Geometry: final body of the model. Coordinates: model frame, mm. A direction names the side the tool comes from. Coordinates: 2 decimals unless noted, no trailing zeros. Order: outer loops, then holes, each group sorted by start corner. A loop starts at its lowest first (then second) coordinate and runs counter-clockwise, first axis right, second up. Notation, with made-up numbers: M 4.5,1 L 13.5,1 A24 ccw 13.5,32 Z; hole C 75.5,89.5 d2. An arc over 180 degrees is marked long. Use CSV: the item, a comma, the result in double quotes. Start each with the question number.
Q1. Section query B-B, the plane x = 19. Output: boundary loops of the cut face in (y, z), and give its area (3 significant figures).
Q2. First-contact query: P1, Ø1.6, axis at y = 1, z = 28, coming from the -X side; P2, Ø1, axis at y = 1, z = -6, coming from the +X side; P3, Ø1.6, axis at y = 1.5, z = -24.5, coming from the +X side. Flat tips, straight axial feed; report the tip coordinate or a pass-through.
Q3. Section query C-C, the plane z = 26. Output: boundary loops of the cut face in (x, y), and give its area (3 significant figures).
Q4. Section query A-A, the plane z = 0. Output: boundary loops of the cut face in (x, y), and give its area (4 significant figures).
Q5. Ray query, probe 1 along X at (y, z) = (5.95, 0); probe 2 along X at (y, z) = (0.45, 25); probe 3 along Z at (x, y) = (1, 1.2). Return the intervals inside material, ascending.
Q6. Access query for faces 1 (the face through (-1.978, 1.972, 2.579)), 2 (the face through (19.529, 1.014, 11.275)). Directions: +Z, -Z, +X, -X, +Y, -Y. A direction counts if a zero-diameter tool reaches every point of the face in a straight line with its end or side. Return the directions, or none.
Q7. Section query D-D, the plane z = -19.5. Output: boundary loops of the cut face in (x, y).
Q8. Mould query, pull axis X, two halves, no side actions, for faces 3 (the face through (-8.378, 1.014, 1.435)), 4 (the face through (-2, 6, 0)), 5 (the face through (-5.37, 3.97, -1.19)), 6 (the face through (36.406, 1.014, -6.603)). Classes: +X half, -X half, draft (parallel to the pull), parting line (faces both ways), or undercut.
from build123d import *

# Parameters (mm, degrees)
CROQUIS1_R              = 40
SALIENTE_EXTRUIR1_DEPTH = 2
CROQUIS2_R              = 5.5
SALIENTE_EXTRUIR2_DEPTH = 4
CROQUIS3_R              = 1.75
CORTAR_EXTRUIR1_DEPTH   = 57.885850613
CROQUIS4_R              = 3.25
CORTAR_EXTRUIR2_DEPTH   = 3.5
CHAFL_N1_SIZE           = 2
CORTAR_EXTRUIR3_DEPTH   = 57.709787515


with BuildPart() as part:
    # Croquis1 → Saliente-Extruir1 (new body)
    with BuildSketch(Plane(origin=(0, 0, 0), x_dir=(1, 0, 0), z_dir=(0, 1, 0))):
        with Locations(Location((0, 0, 0), (0, 0, 270))):
            Circle(CROQUIS1_R)
    extrude(amount=SALIENTE_EXTRUIR1_DEPTH)

    # Croquis2 → Saliente-Extruir2 (add)
    with BuildSketch(Plane(origin=(0, 2, 0), x_dir=(1, 0, 0), z_dir=(0, 1, 0))):
        with Locations(Location((0, 0, 0), (0, 0, 270))):
            Circle(CROQUIS2_R)
    extrude(amount=SALIENTE_EXTRUIR2_DEPTH)

    # Croquis3 → Cortar-Extruir1 (cut, through all)
    with BuildSketch(Plane(origin=(0, 6, 0), x_dir=(1, 0, 0), z_dir=(0, 1, 0))):
        with Locations(Location((0, 0, 0), (0, 0, 270))):
            Circle(CROQUIS3_R)
    extrude(amount=-CORTAR_EXTRUIR1_DEPTH, mode=Mode.SUBTRACT)

    # Croquis4 → Cortar-Extruir2 (cut)
    with BuildSketch(Plane(origin=(0, 0, 0), x_dir=(-1, 0, 0), z_dir=(0, -1, 0))):
        with Locations(Location((0, 0, 0), (0, 0, 90))):
            Circle(CROQUIS4_R)
    extrude(amount=-CORTAR_EXTRUIR2_DEPTH, mode=Mode.SUBTRACT)

    # Chaflán1
    # the kernel refuses this chamfer: 2 mm, written as the material it takes off along each edge
    with BuildSketch(Plane(origin=(0, 3.5, 0), x_dir=(0, 0, 1), z_dir=(-1, 0, 0))) as chafl_n1_piece_1_section:
        Polygon((1.75 + CHAFL_N1_SIZE, 0), (1.75, CHAFL_N1_SIZE), (1.75, 0), align=None)
    chafl_n1_piece_1 = revolve(axis=Axis((0, 3.5, 0), (0, 1, 0)), mode=Mode.PRIVATE)
    chafl_n1_piece_1 = chafl_n1_piece_1 & Plane(origin=(0, 4.756379489, 0), x_dir=(0, 0, -1), z_dir=(0, -1, 0)) * Cylinder(3.25, 15, mode=Mode.PRIVATE)
    add(chafl_n1_piece_1, mode=Mode.SUBTRACT)

    # Croquis5 → Cortar-Extruir3 (cut, through all)
    with BuildSketch(Plane(origin=(0, 2, 0), x_dir=(1, 0, 0), z_dir=(0, 1, 0))):
        with BuildLine():
            Line((0, 8.5), (0, 37))
            ThreePointArc((0, 37), (12.654745303, 34.768626969), (23.783141558, 28.343644395))
            Line((23.783141558, 28.343644395), (5.463694682, 6.511377767))
            ThreePointArc((5.463694682, 6.511377767), (2.907171218, 7.987387277), (0, 8.5))
        make_face()
        with BuildLine():
            Line((7.361215932, 4.25), (32.04293994, 18.5))
            ThreePointArc((32.04293994, 18.5), (36.437886861, 6.424982574), (36.437886861, -6.424982574))
            Line((36.437886861, -6.424982574), (8.370865901, -1.47600951))
            ThreePointArc((8.370865901, -1.47600951), (8.370865901, 1.47600951), (7.361215932, 4.25))
        make_face()
        with BuildLine():
            Line((7.361215932, -4.25), (32.04293994, -18.5))
            ThreePointArc((32.04293994, -18.5), (23.783141558, -28.343644395), (12.654745303, -34.768626969))
            Line((12.654745303, -34.768626969), (2.907171218, -7.987387277))
            ThreePointArc((2.907171218, -7.987387277), (5.463694682, -6.511377767), (7.361215932, -4.25))
        make_face()
        with BuildLine():
            Line((0, -8.5), (0, -37))
            ThreePointArc((0, -37), (-12.654745303, -34.768626969), (-23.783141558, -28.343644395))
            Line((-23.783141558, -28.343644395), (-5.463694682, -6.511377767))
            ThreePointArc((-5.463694682, -6.511377767), (-2.907171218, -7.987387277), (0, -8.5))
        make_face()
        with BuildLine():
            Line((-7.361215932, -4.25), (-32.04293994, -18.5))
            ThreePointArc((-32.04293994, -18.5), (-36.437886861, -6.424982574), (-36.437886861, 6.424982574))
            Line((-36.437886861, 6.424982574), (-8.370865901, 1.47600951))
            ThreePointArc((-8.370865901, 1.47600951), (-8.370865901, -1.47600951), (-7.361215932, -4.25))
        make_face()
        with BuildLine():
            Line((-7.361215932, 4.25), (-32.04293994, 18.5))
            ThreePointArc((-32.04293994, 18.5), (-23.783141558, 28.343644395), (-12.654745303, 34.768626969))
            Line((-12.654745303, 34.768626969), (-2.907171218, 7.987387277))
            ThreePointArc((-2.907171218, 7.987387277), (-5.463694682, 6.511377767), (-7.361215932, 4.25))
        make_face()
    extrude(amount=-CORTAR_EXTRUIR3_DEPTH, mode=Mode.SUBTRACT)


solid = part.part
Responses:
1,outline,"M 0,-35.2 L 2,-35.2 L 2,-31.75 L 0,-31.75 Z; M 0,-22.64 L 2,-22.64 L 2,-10.97 L 0,-10.97 Z; M 0,3.35 L 2,3.35 L 2,10.97 L 0,10.97 Z; M 0,31.75 L 2,31.75 L 2,35.2 L 0,35.2 Z"
1,area,"52.4 mm²"
2,P1,"stops at x = -29.33"
2,P2,"stops at x = 39.62"
2,P3,"stops at x = 32.22"
3,outline,"M -30.4,0 L -21.82,0 L -21.82,2 L -30.4,2 Z; M 0,0 L 9.46,0 L 9.46,2 L 0,2 Z; M 26.32,0 L 30.4,0 L 30.4,2 L 26.32,2 Z"
3,area,"44.2 mm²"
4,outline,"M -40,0 L -37,0 L -37,2 L -40,2 Z; M -8.5,0 L -3.25,0 L -3.25,4 L -1.75,5.5 L -1.75,6 L -5.5,6 L -5.5,2 L -8.5,2 Z; M 1.75,5.5 L 3.25,4 L 3.25,0 L 8.5,0 L 8.5,2 L 5.5,2 L 5.5,6 L 1.75,6 Z; M 37,0 L 40,0 L 40,2 L 37,2 Z"
4,area,"54.75 mm²"
5,probe 1,"x = -5.5 to -1.75, 1.75 to 5.5"
5,probe 2,"x = -31.22 to -20.98, 0 to 9.1, 27.28 to 31.22"
5,probe 3,"z = -39.99 to -36.99, -8.44 to -3.09, 3.09 to 39.99"
6,face 1,"-Y"
6,face 2,"+Y, -Y"
7,outline,"M -34.92,0 L -31.44,0 L -31.44,2 L -34.92,2 Z; M -7.1,0 L 0,0 L 0,2 L -7.1,2 Z; M 16.36,0 L 34.92,0 L 34.92,2 L 16.36,2 Z"
8,face 3,"undercut"
8,face 4,"draft"
8,face 5,"parting line"
8,face 6,"undercut"
